The listing builds one solid part. Answer for the finished solid, in the listing's coordinates (mm). Round coordinates to 2 decimals unless told otherwise and drop trailing zeros. Write each loop counter-clockwise with the first axis right and the second up, starting at its lowest first coordinate (ties: lowest second). Pieces come first, ordered by that corner, then holes.
from build123d import *

# Parameters (mm, degrees)
ESQUISSE1_W             = 200
ESQUISSE1_H             = 100
ESQUISSE1_R             = 2
ESQUISSE1_R_2           = 1.6
BOSS_EXTRU_1_DEPTH      = 4
ENL_V_MAT_EXTRU_1_DEPTH = 10
BOSS_EXTRU_2_DEPTH      = 2
ESQUISSE4_W             = 200
ESQUISSE4_H             = 4.471345155
BOSS_EXTRU_3_DEPTH      = 2
CHANFREIN1_SIZE         = 5


with BuildPart() as part:
    # Esquisse1 → Boss.-Extru.1 (new body)
    with BuildSketch(Plane(origin=(0, 0, 0), x_dir=(1, 0, 0), z_dir=(0, 1, 0))):
        Rectangle(ESQUISSE1_W, ESQUISSE1_H)
        with Locations(Location((-92, 42, 0), (0, 0, 270))):
            Circle(ESQUISSE1_R, mode=Mode.SUBTRACT)
        with Locations(Location((92, 42, 0), (0, 0, 90))):
            Circle(ESQUISSE1_R, mode=Mode.SUBTRACT)
        with Locations(Location((92, -42, 0), (0, 0, 270))):
            Circle(ESQUISSE1_R, mode=Mode.SUBTRACT)
        with Locations(Location((-92, -42, 0), (0, 0, 90))):
            Circle(ESQUISSE1_R, mode=Mode.SUBTRACT)
        with Locations(Location((-6.5, -15, 0), (0, 0, 270))):
            Circle(ESQUISSE1_R, mode=Mode.SUBTRACT)
        with Locations(Location((20, 0, 0), (0, 0, 270))):
            Circle(ESQUISSE1_R, mode=Mode.SUBTRACT)
        with Locations(Location((-6.5, 15, 0), (0, 0, 90))):
            Circle(ESQUISSE1_R, mode=Mode.SUBTRACT)
        with Locations(Location((-33.1, -20.3, 0), (0, 0, 270))):
            Circle(ESQUISSE1_R_2, mode=Mode.SUBTRACT)
        with Locations(Location((-33.1, 7.6, 0), (0, 0, 270))):
            Circle(ESQUISSE1_R_2, mode=Mode.SUBTRACT)
        with Locations(Location((-85, -25, 0), (0, 0, 270))):
            Circle(ESQUISSE1_R_2, mode=Mode.SUBTRACT)
        with Locations(Location((-83.8, 22.7, 0), (0, 0, 270))):
            Circle(ESQUISSE1_R_2, mode=Mode.SUBTRACT)
    extrude(amount=BOSS_EXTRU_1_DEPTH)

    # Esquisse2 → Enlèv. mat.-Extru.1 (cut)
    with BuildSketch(Plane(origin=(0, 4, 0), x_dir=(1, 0, 0), z_dir=(0, 1, 0))):
        with BuildLine():
            Line((-71.12395108, 33.267340446), (-71.12395108, -35.262942493))
            add(Edge.make_bspline(
                [(-71.12395108, -35.262942493), (-71.80811413, -39.025609189), (-68.179899303, -39.50320708)],
                knots=[0, 0, 0, 1, 1, 1], degree=2))
            Line((-68.179899303, -39.50320708), (-48.41260505, -39.50320708))
            add(Edge.make_bspline(
                [(-45.119156215, -35.262942493), (-44.797316754, -39.038148597), (-48.41260505, -39.50320708)],
                knots=[0, 0, 0, 1, 1, 1], degree=2))
            Line((-45.119156215, -35.262942493), (-45.119156215, 33.267340446))
            add(Edge.make_bspline(
                [(-48.41260505, 36.799015417), (-44.987803153, 36.784833779), (-45.119156215, 33.267340446)],
                knots=[0, 0, 0, 1, 1, 1], degree=2))
            Line((-48.41260505, 36.799015417), (-68.179899303, 36.799015417))
            add(Edge.make_bspline(
                [(-68.179899303, 36.799015417), (-71.625685069, 36.783683635), (-71.12395108, 33.267340446)],
                knots=[0, 0, 0, 1, 1, 1], degree=2))
        make_face()
        with BuildLine():
            Line((29.185631994, 32.76936094), (29.185631994, -35.760921998))
            add(Edge.make_bspline(
                [(29.185631994, -35.760921998), (28.501468944, -39.523588695), (32.129683771, -40.001186586)],
                knots=[0, 0, 0, 1, 1, 1], degree=2))
            Line((32.129683771, -40.001186586), (78.655845139, -40.001186586))
            add(Edge.make_bspline(
                [(82.138089103, -35.760921998), (82.221370803, -39.504216764), (78.655845139, -40.001186586)],
                knots=[0, 0, 0, 1, 1, 1], degree=2))
            Line((82.138089103, -35.760921998), (82.138089103, 32.76936094))
            add(Edge.make_bspline(
                [(78.655845139, 36.301035912), (82.034782777, 36.251456851), (82.138089103, 32.76936094)],
                knots=[0, 0, 0, 1, 1, 1], degree=2))
            Line((78.655845139, 36.301035912), (32.129683771, 36.301035912))
            add(Edge.make_bspline(
                [(32.129683771, 36.301035912), (28.683898005, 36.28570413), (29.185631994, 32.76936094)],
                knots=[0, 0, 0, 1, 1, 1], degree=2))
        make_face()
    extrude(amount=-ENL_V_MAT_EXTRU_1_DEPTH, mode=Mode.SUBTRACT)

    # Esquisse3 → Boss.-Extru.2 (add)
    with BuildSketch(Plane.XZ):
        Polygon((-100, 50), (-100, 61.471345155), (0, 61.471345155), (100, 61.471345155), (100, 50), align=None)
    extrude(amount=-BOSS_EXTRU_2_DEPTH)

    # Esquisse4 → Boss.-Extru.3 (add)
    with BuildSketch(Plane(origin=(0, 2, 0), x_dir=(1, 0, 0), z_dir=(0, 1, 0))):
        with Locations((0, -59.235672577)):
            Rectangle(ESQUISSE4_W, ESQUISSE4_H)
    extrude(amount=BOSS_EXTRU_3_DEPTH)

    # Chanfrein1
    chanfrein1_edges = [part.edges().sort_by_distance(p)[0] for p in [
        (-100, 2, -50),
        (100, 2, -50),
    ]]
    chamfer(chanfrein1_edges, length=CHANFREIN1_SIZE)


solid = part.part
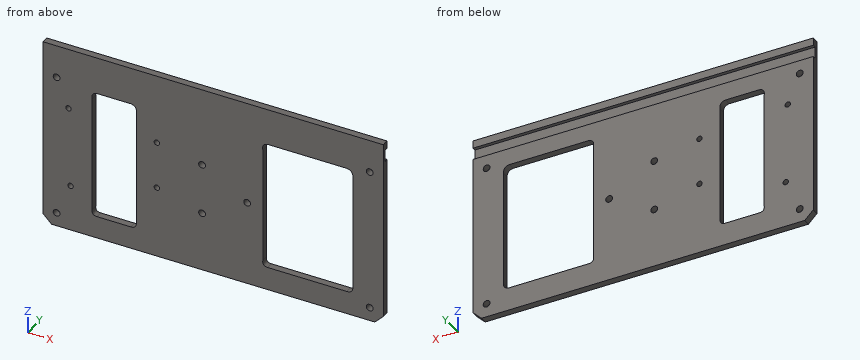
1. Section A-A on x = 20 is taken. Determine the outline of the cut face in (y, z), plus the area to 3 significant figures.
Geometry says:
outline: (0, -50) - (4, -50) - (4, -2) - (0, -2) - close; (0, 2) - (4, 2) - (4, 50) - (2, 50) - (2, 57) - (4, 57) - (4, 61.47) - (0, 61.47) - close
area: 416 mm2
2. Section C-C on x = 92 is taken. Determine the outline of the cut face in (y, z), plus the area to 3 significant figures.
Geometry says:
outline: (0, -50) - (4, -50) - (4, -44) - (0, -44) - close; (0, -40) - (4, -40) - (4, 40) - (0, 40) - close; (0, 44) - (4, 44) - (4, 50) - (2, 50) - (2, 57) - (4, 57) - (4, 61.47) - (0, 61.47) - close
area: 400 mm2
3. Given pin 1 (6.5 mm diameter, centred on x = 92, z = -42, fed in from +Y), flat-ended and moving along its own axis, determine where the tip first touches the part or whether it passes through.
Geometry says:
pin 1: stops at y = 4
4. Section D-D on z = 0 is taken. Determine the outline of the cut face in (x, y).
Geometry says:
outline: (-100, 0) - (-71.12, 0) - (-71.12, 4) - (-100, 4) - close; (-45.12, 0) - (18, 0) - (18, 4) - (-45.12, 4) - close; (22, 0) - (29.19, 0) - (29.19, 4) - (22, 4) - close; (82.14, 0) - (100, 0) - (100, 4) - (82.14, 4) - close
5. Section B-B on z = -29 is taken. Determine the outline of the cut face in (x, y).
Geometry says:
outline: (-100, 0) - (-71.12, 0) - (-71.12, 4) - (-100, 4) - close; (-45.12, 0) - (29.19, 0) - (29.19, 4) - (-45.12, 4) - close; (82.14, 0) - (100, 0) - (100, 4) - (82.14, 4) - close
6. Straight lines are drawn through the part: line 1 along X through (y, z) = (0.95, 15); line 2 along X through (y, z) = (1.6, 25); line 3 along X through (y, z) = (2.55, 22). For each, find the intervals that lie inside material, in ascending order.
Geometry says:
line 1: x = -100 to -71.12, -45.12 to -8.5, -4.5 to 29.19, 82.14 to 100
line 2: x = -100 to -86.6, -83.4 to -71.12, -45.12 to 29.19, 82.14 to 100
line 3: x = -100 to -71.12, -45.12 to 29.19, 82.14 to 100
